Check sheet for the modelled part. Datum: model origin and axes. Units: mm. A direction names the side the tool comes from. Round coordinates to 2 decimals unless told otherwise and drop trailing zeros. Write each loop counter-clockwise with the first axis right and the second up, starting at its lowest first coordinate (ties: lowest second). Pieces come first, ordered by that corner, then holes.
Item 1: Section check A-A, the plane x = 0. Record the cut outline in (y, z).
Item 2: Release check for a two-part mould opening along Z. For faces 3 (the flat face through (39.751, -6, -1)), 4 (the flat face through (-1, -6, 58.801)), 5 (the cylindrical face through (-22.79, -6.44, 42.77)), 6 (the flat face through (-1, -6, -58.801)) record: pulls with the +Z half, pulls with the -Z half, needs draft (parallel to the pull), parting line crosses it, or undercut.
Item 3: Depth check by flat-ended pin: pin 1 (4 mm diameter, centred on x = -24, z = 24.5, fed in from +Y); pin 2 (4 mm diameter, centred on y = 14, z = 17, fed in from +X); pin 3 (2 mm diameter, centred on x = -23.749, z = 41.275, fed in from +Y); pin 4 (1.5 mm diameter, centred on x = 19, y = 26.5, fed in from +Z). Enter the tip coordinate at first touch or a pass-through.
Item 4: Set-up check for faces 1 (the flat face through (0, 36.322, -26)), 2 (the cylindrical face through (-20.23, 17.91, 32.28)): record each of +Z, -Z, +X, -X, +Y, -Y from which the full face is reachable in a straight line by a thin tool's end or side.
Item 5: Section check D-D, the plane x = -8. Record the cut outline in (y, z).
Item 6: Material ranges on line 1 along Y through (x, z) = (-29, 20); line 2 along Z through (x, y) = (-16.5, 20); line 3 along X through (y, z) = (-7, -40), recorded low to high.
Item 7: Section check C-C, the plane y = 29. Record the cut outline in (x, z), plus the area to 3 significant figures.
Item 8: Section check B-B, the plane z = 12. Record the cut outline in (x, y), plus the area to 3 significant figures.
from build123d import *

# Parameters (mm, degrees)
F0_W     = 79.502
F0_H     = 117.602
F1_DEPTH = 12.7
F2_R     = 1.778
F3_DEPTH = 12.701
F4_R     = 21.209
F5_DEPTH = 36.322


with BuildPart() as f1:
    # F0 (on Front) → F1 (new body)
    with BuildSketch(Plane.XZ):
        Rectangle(F0_W, F0_H)
    extrude(amount=F1_DEPTH)

    # F2 (on face) → F3 (cut, through all)
    with BuildSketch(Plane.XZ.offset(12.7)):
        with Locations((-23.749, 41.275)):
            Circle(F2_R)
        with Locations((23.749, 41.275)):
            Circle(F2_R)
        with Locations((-23.749, -41.275)):
            Circle(F2_R)
        with Locations((23.749, -41.275)):
            Circle(F2_R)
    extrude(amount=-F3_DEPTH, mode=Mode.SUBTRACT)

    # F4 (on face) → F5 (join)
    with BuildSketch(Plane(origin=(0, 0, 0), x_dir=(-1, 0, 0), z_dir=(0, 1, 0))):
        with Locations((0, 25.908)):
            Circle(F4_R)
        with Locations((0, -25.908)):
            Circle(F4_R)
    extrude(amount=F5_DEPTH)


solid = f1.part
Values found:
1. outline: (-12.7, -58.8) - (0, -58.8) - (0, -47.12) - (36.32, -47.12) - (36.32, -4.7) - (0, -4.7) - (0, 4.7) - (36.32, 4.7) - (36.32, 47.12) - (0, 47.12) - (0, 58.8) - (-12.7, 58.8) - close
2. face 3: needs draft
2. face 4: pulls with the +Z half
2. face 5: undercut
2. face 6: pulls with the -Z half
3. pin 1: stops at y = 0
3. pin 2: stops at x = 20.05
3. pin 3: passes through
3. pin 4: stops at z = 36.71
4. face 1: +Z, -Z, +X, -X, +Y
4. face 2: +Y
5. outline: (-12.7, -58.8) - (0, -58.8) - (0, -45.55) - (36.32, -45.55) - (36.32, -6.27) - (0, -6.27) - (0, 6.27) - (36.32, 6.27) - (36.32, 45.55) - (0, 45.55) - (0, 58.8) - (-12.7, 58.8) - close
6. line 1: y = -12.7 to 0
6. line 2: z = -39.23 to -12.58, 12.58 to 39.23
6. line 3: x = -39.75 to -24.99, -22.51 to 22.51, 24.99 to 39.75
7. outline: circle Ø42.42 at (0, -25.91); circle Ø42.42 at (0, 25.91)
7. area: 2,830 mm2
8. outline: (-39.75, -12.7) - (39.75, -12.7) - (39.75, 0) - (16.01, 0) - (16.01, 36.32) - (-16.01, 36.32) - (-16.01, 0) - (-39.75, 0) - close
8. area: 2,170 mm2
